from build123d import *

# Parameters (mm, degrees)
F1_DEPTH = 609.6
F3_DEPTH = 38.101
F4_R     = 4.7625
F5_DEPTH = 38.101


with BuildPart() as f1:
    # F0 (on Right) → F1 (new body)
    with BuildSketch(Plane.YZ):
        Polygon((0, 3.175), (0, 0), (38.1, 0), (38.1, 38.1), (34.925, 38.1), (34.925, 3.175), align=None)
    extrude(amount=F1_DEPTH)

    # F2 (on face) → F3 (cut, through all)
    with BuildSketch(Plane(origin=(0, 38.1, 0), x_dir=(-1, 0, 0), z_dir=(0, 1, 0))):
        Polygon((-571.5, 0), (-609.6, 38.1), (-609.6, 0), align=None)
        Polygon((0, 0), (0, 38.1), (-38.1, 0), align=None)
    extrude(amount=-F3_DEPTH, mode=Mode.SUBTRACT)

    # F4 (on face) → F5 (cut, through all)
    with BuildSketch(Plane(origin=(0, 38.1, 0), x_dir=(-1, 0, 0), z_dir=(0, 1, 0))):
        with Locations((-45.990768, 19.05)):
            Circle(F4_R)
        with Locations((-563.609232, 19.05)):
            Circle(F4_R)
    extrude(amount=-F5_DEPTH, mode=Mode.SUBTRACT)


solid = f1.part
Build history of the part. All positions in model axes, mm. A direction names the side the tool comes from. Round coordinates to 2 decimals unless told otherwise and drop trailing zeros. Loops run counter-clockwise (first coordinate to the right, second up) from the corner with the lowest first, then second, coordinate; pieces in that order, holes last. Notation, with made-up numbers: (9.25, -12) -> (45.25, -12) arc R7 ccw to (45.25, -4) -> close; hole circle Ø6 at (30.5, -21). An arc over 180 degrees is marked (long way). One line per item, written item: value. Start each with the question number.
Q1. 3-axis set-ups, long thin cutter, end or side, ignore diameter. For faces 4 (the face through (301, 18, 3.175)), 5 (the face through (301, 19, 0)): which of +Z, -Z, +X, -X, +Y, -Y reach the whole face in a straight line?
Q2. Cut at A-A on x = 175.5. List the corners of the cut face in (y, z) (3 decimals), plus the area to 3 significant figures.
Q3. Two-plate mould, pull along Z, no slides. Class faces 1 (the face through (301, 34.925, 21)), 2 (the face through (27.4, 36.1, 10.7)), 3 (the face through (43.43, 36.535, 23.066)): released by +Z, released by -Z, zero draft, split by the parting line, or undercut.
Q4. Cut at C-C on y = 26. List the corners of the cut face in (x, z) (3 decimals), plus the area to 3 significant figures.
Q5. Probe line 1 along Z through (x, y) = (312.5, 15.5) (3 decimals); line 2 along Y through (x, z) = (239.5, 27) (3 decimals); line 3 along X through (y, z) = (36, 19). List the from-to ranges inside material, lowest first.
Q6. Drop flat-ended pins along their axis: pin 1 Ø1 at (x, y) = (181.5, 14.5) entering from +Z (3 decimals); pin 2 Ø6 at (x, z) = (135.5, 23.5) entering from -Y (3 decimals). Give the stop position or say it passes through.
Q7. Cut at B-B on z = 33. List the corners of the cut face in (x, y) (3 decimals).
Computed:
1. face 4: +Z, +X, -X, -Y
1. face 5: -Z, +X, -X, +Y, -Y
2. outline: (0, 0) -> (38.1, 0) -> (38.1, 38.1) -> (34.925, 38.1) -> (34.925, 3.175) -> (0, 3.175) -> close
2. area: 232 mm²
3. face 1: zero draft
3. face 2: released by -Z
3. face 3: undercut
4. outline: (34.925, 3.175) -> (38.1, 0) -> (571.5, 0) -> (574.675, 3.175) -> close
4. area: 1,700 mm²
5. line 1: 0 to 3.175
5. line 2: 34.925 to 38.1
5. line 3: 19.1 to 41.23, 50.75 to 558.85, 568.37 to 590.5
6. pin 1: z = 3.175
6. pin 2: y = 34.925
7. outline: (5.1, 34.925) -> (604.5, 34.925) -> (604.5, 38.1) -> (5.1, 38.1) -> close
